Verification items for the finished model (mm, model axes). A direction names the side the tool comes from. Give positions to 0.01 mm unless a question says otherwise; leave off trailing zeros. Order: outer loops, then holes, each group sorted by start corner. A loop starts at its lowest first (then second) coordinate and runs counter-clockwise, first axis right, second up. Notation, with made-up numbers: (8.25, 66.5) - (50.25, 66.5) arc R18 ccw to (50.25, 73.5) - close; hole circle Ø3 at (54, -34). An arc over 180 degrees is marked (long way). Answer as a JSON object with one key per item and string values.
```python
from build123d import *

# Parameters (mm, degrees)
ESQUISSE1_W                = 30
ESQUISSE1_H                = 700
BOSS_EXTRU_1_DEPTH         = 30
ESQUISSE2_W                = 30
ESQUISSE2_H                = 30
ESQUISSE2_H_2              = 2
BOSS_EXTRU_2_DEPTH         = 30
ESQUISSE3_W                = 26
ESQUISSE3_H                = 26
ENL_V_MAT_EXTRU_1_DEPTH    = 30
R_P_TITION_LIN_AIRE2_COUNT = 3
R_P_TITION_LIN_AIRE2_PITCH = 670
ESQUISSE4_W                = 26
ESQUISSE4_H                = 26
ENL_V_MAT_EXTRU_2_DEPTH    = 703.726831706
ESQUISSE5_R                = 3.05
ENL_V_MAT_EXTRU_3_DEPTH    = 703.726831706
ESQUISSE7_R                = 7.05
ENL_V_MAT_EXTRU_4_DEPTH    = 28


with BuildPart() as part:
    # Esquisse1 → Boss.-Extru.1 (new body)
    with BuildSketch(Plane.XY):
        Rectangle(ESQUISSE1_W, ESQUISSE1_H)
    extrude(amount=BOSS_EXTRU_1_DEPTH)

    # Esquisse2 → Boss.-Extru.2 (add)
    with BuildSketch(Plane.XY.offset(30)):
        with Locations((0, 335)):
            Rectangle(ESQUISSE2_W, ESQUISSE2_H)
        with Locations((0, -335)):
            Rectangle(ESQUISSE2_W, ESQUISSE2_H)
        Rectangle(ESQUISSE2_W, ESQUISSE2_H_2)
    extrude(amount=BOSS_EXTRU_2_DEPTH)

    # Esquisse3 → Enlèv. mat.-Extru.1 (cut)
    with BuildSketch(Plane.XY.offset(60)):
        with Locations((0, 335)):
            Rectangle(ESQUISSE3_W, ESQUISSE3_H)
    enl_v_mat_extru_1 = extrude(amount=-ENL_V_MAT_EXTRU_1_DEPTH, mode=Mode.SUBTRACT)

    # Répétition linéaire2: Enlèv. mat.-Extru.1 ×3
    with Locations(*[(0, -i * R_P_TITION_LIN_AIRE2_PITCH, 0) for i in range(1, R_P_TITION_LIN_AIRE2_COUNT)]):
        add(enl_v_mat_extru_1, mode=Mode.SUBTRACT)

    # Esquisse4 → Enlèv. mat.-Extru.2 (cut, through all)
    with BuildSketch(Plane(origin=(0, -350, 0), x_dir=(-1, 0, 0), z_dir=(0, -1, 0))):
        with Locations((0, -15)):
            Rectangle(ESQUISSE4_W, ESQUISSE4_H)
    extrude(amount=-ENL_V_MAT_EXTRU_2_DEPTH, mode=Mode.SUBTRACT)

    # Esquisse5 → Enlèv. mat.-Extru.3 (cut, through all)
    with BuildSketch(Plane(origin=(0, -350, 0), x_dir=(-1, 0, 0), z_dir=(0, -1, 0))):
        with Locations(Location((10, -45, 0), (0, 0, 90))):
            Circle(ESQUISSE5_R)
        with Locations(Location((-10, -45, 0), (0, 0, 90))):
            Circle(ESQUISSE5_R)
    extrude(amount=-ENL_V_MAT_EXTRU_3_DEPTH, mode=Mode.SUBTRACT)

    # Esquisse7 → Enlèv. mat.-Extru.4 (cut)
    with BuildSketch(Plane(origin=(0, 0, 0), x_dir=(-1, 0, 0), z_dir=(0, 0, -1))):
        Circle(ESQUISSE7_R)
    extrude(amount=-ENL_V_MAT_EXTRU_4_DEPTH, mode=Mode.SUBTRACT)


solid = part.part
```
(1) Release check for a two-part mould opening along X. For faces 1 (the flat face through (-15, -5, 16)), 2 (the flat face through (0, -158, 30)), 3 (the flat face through (15, -5, 16)), 4 (the flat face through (-13, -5, 15)) record: pulls with the +X half, pulls with the -X half, needs draft (parallel to the pull), parting line crosses it, or undercut.
Computed values:
{"face 1": "pulls with the -X half", "face 2": "needs draft", "face 3": "pulls with the +X half", "face 4": "undercut"}
(2) Gauge pin test, flat end, axial feed: pin 1 Ø1 at (x, y) = (-10.5, 151.5) entering from +Z. Record the tip position at first contact, or that the pin passes through.
Computed values:
{"pin 1": "stops at z = 30"}
(3) Material ranges on line 1 along X through (y, z) = (0.4, 45); line 2 along Y through (x, z) = (4.5, 45.5); line 3 along Y through (x, z) = (13.5, 35), recorded low to high. Write a range as [from, to].
Computed values:
{"line 1": "x = [-15, -13.05], [-6.95, 6.95], [13.05, 15]", "line 2": "y = [-350, -348], [-322, -320], [-1, 1], [320, 322], [348, 350]", "line 3": "y = [-350, -320], [-1, 1], [320, 350]"}
(4) Section check B-B (y = -36). Record the cut outline in (x, z), then the cut area to 3 significant figures.
Computed values:
{"outline": "(-15, 0) - (15, 0) - (15, 30) - (-15, 30) - close; hole (-13, 2) - (13, 2) - (13, 28) - (-13, 28) - close", "area": "224 mm²"}
(5) Access from +Z, -Z, +X, -X, +Y, -Y to the whole of each face (thin tool, end or side, straight path). Record for faces 5 (the flat face through (6, -5, 2)), 6 (the flat face through (0, 1, 45)), 7 (the flat face through (-13, 335, 37)), 8 (the flat face through (0, 350, 36)), 9 (the cylindrical face through (-3.253, -6.255, 0.986)).
Computed values:
{"face 5": "+Y, -Y", "face 6": "+Z, +X, -X", "face 7": "+Z", "face 8": "+Z, -Z, +X, -X, +Y", "face 9": "-Z"}
(6) Section check A-A (z = 10.5). Record the cut outline in (x, y).
Computed values:
{"outline": "(-15, -350) - (-13, -350) - (-13, 350) - (-15, 350) - close; (13, -350) - (15, -350) - (15, 350) - (13, 350) - close"}
